Geometry check sheet. Reference: the model listing, model coordinates, mm. A direction names the side the tool comes from. Coordinates: 2 decimals unless noted, no trailing zeros. Write each loop counter-clockwise with the first axis right and the second up, starting at its lowest first coordinate (ties: lowest second). Pieces come first, ordered by that corner, then holes. Notation, with made-up numbers: (79.25, 72.25) -> (83.25, 72.25) arc R30 ccw to (83.25, 110.25) -> close; hole circle Ø11 at (59, 15.5). An arc over 180 degrees is marked (long way). Answer as CSV lines item,"result".
```python
from build123d import *

# Parameters (mm, degrees)
SKETCH_2_W        = 80
SKETCH_2_H        = 100
EXTRUDE_1_DEPTH   = 100
OTHER_START       = 98.38699101
OTHER_1_OUTLINE_W = 92
OTHER_1_OUTLINE_H = 80
OTHER_1_DEPTH     = 35.77708764
SHELL_3_T         = -3


with BuildPart() as part:
    # 草图2 → 凸台-拉伸1 (new body)
    with BuildSketch(Plane(origin=(0, 0, 0), x_dir=(0, 0, -1), z_dir=(1, 0, 0))):
        with Locations((40, -50)):
            Rectangle(SKETCH_2_W, SKETCH_2_H)
    extrude(amount=EXTRUDE_1_DEPTH)

    # 边界-切除1: read off the stored shape, not the designer's step
    # 边界-切除1 outline → 边界-切除1 (cut)
    with BuildSketch(Plane(origin=(0, 0, 0), x_dir=(0.8944271909999159, 0.44721359549995804, 0), z_dir=(0.447213595499958, -0.894427190999916, 0)).offset(OTHER_START)):
        with Locations((18, -40)):
            Rectangle(OTHER_1_OUTLINE_W, OTHER_1_OUTLINE_H)
    extrude(amount=OTHER_1_DEPTH, mode=Mode.SUBTRACT)

    # 抽壳3
    shell_3_openings = [part.faces().sort_by_distance(p)[0] for p in [
        (10, -100, -40),
        (50, 0, -40),
    ]]
    offset(amount=SHELL_3_T, openings=shell_3_openings, kind=Kind.INTERSECTION)


solid = part.part
```
Item 1: Release check for a two-part mould opening along X. For faces 1 (the flat face through (0, -49, -39)), 2 (the flat face through (49, -40, -77)), 3 (the flat face through (50, 0, -1)) record: +X half, -X half, draft (parallel to the pull), parting line (faces both ways), or undercut.
Responses:
face 1,"-X half"
face 2,"undercut"
face 3,"draft"
Item 2: Depth check by flat-ended pin: pin 1 Ø1 at (x, z) = (48, -13.5) entering from -Y; pin 2 Ø4 at (x, z) = (58, -16) entering from +Y; pin 3 Ø4 at (x, z) = (69, -12) entering from +Y. Enter the tip coordinate at first touch or a pass-through.
Responses:
pin 1,"stops at y = -86.25"
pin 2,"stops at y = -76.65"
pin 3,"stops at y = -71.15"
Item 3: Cross-section at A-A, the plane z = -36. Record the cut outline in (x, y).
Responses:
outline,"(0, -100) -> (3, -100) -> (3, 0) -> (0, 0) -> close; (13.29, -100) -> (20, -100) -> (100, -60) -> (100, 0) -> (97, 0) -> (97, -58.15) -> close"
Item 4: Cross-section at C-C, the plane x = 70. Record the cut outline in (y, z), plus the area to 3 significant figures.
Responses:
outline,"(-75, -80) -> (0, -80) -> (0, -77) -> (-71.65, -77) -> (-71.65, -3) -> (0, -3) -> (0, 0) -> (-75, 0) -> close"
area,"698 mm2"
Item 5: Cross-section at B-B, the plane y = -45. Record the cut outline in (x, z), plus the area to 3 significant figures.
Responses:
outline,"(0, -80) -> (100, -80) -> (100, 0) -> (0, 0) -> close; hole (3, -77) -> (97, -77) -> (97, -3) -> (3, -3) -> close"
area,"1,040 mm2"
Item 6: Cross-section at D-D, the plane y = -86.5. Record the cut outline in (x, z), plus the area to 3 significant figures.
Responses:
outline,"(0, -80) -> (47, -80) -> (47, 0) -> (0, 0) -> close; hole (3, -77) -> (40.29, -77) -> (40.29, -3) -> (3, -3) -> close"
area,"1,000 mm2"
Item 7: Set-up check for faces 4 (the flat face through (49, -40, -3)), 5 (the flat face through (49, -40, -80)), 6 (the flat face through (3, -49, -39)): record each of +Z, -Z, +X, -X, +Y, -Y from which the full face is reachable in a straight line by a thin tool's end or side.
Responses:
face 4,"+Y"
face 5,"-Z, +X, -X, +Y, -Y"
face 6,"+Y, -Y"
Item 8: Thickness scan on probe 1 along Z at (x, y) = (47, -52.5); probe 2 along X at (y, z) = (-16, -52); probe 3 along X at (y, z) = (-88.5, -76). Record the ranges inside material, lowest first.
Responses:
probe 1,"z = -80 to -77, -3 to 0"
probe 2,"x = 0 to 3, 97 to 100"
probe 3,"x = 0 to 3, 36.29 to 43"
